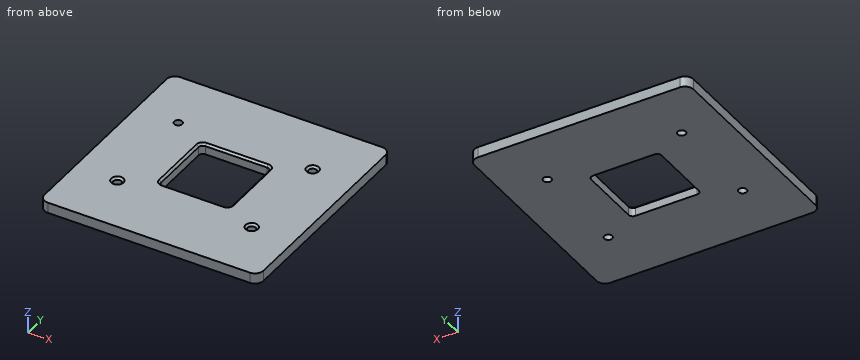
```python
from build123d import *

# Parameters (mm, degrees)
CYLINDER006_R     = 1.9
CYLINDER006_DEPTH = 5
CYLINDER007_R     = 1.9
CYLINDER007_DEPTH = 5
CYLINDER008_R     = 1.9
CYLINDER008_DEPTH = 5
CYLINDER005_R     = 1.9
CYLINDER005_DEPTH = 5
BOX009_W          = 33
BOX009_H          = 33
BOX009_DEPTH      = 5
BOX010_W          = 72
BOX010_H          = 72
BOX010_DEPTH      = 5
FILLET002_R       = 2
FILLET003_R       = 4
CHAMFER001_SIZE   = 1
BOX013_W          = 69.4
BOX013_H          = 69.4
BOX013_DEPTH      = 5
BOX012_W          = 103
BOX012_H          = 103
BOX012_DEPTH      = 5
FILLET005_R       = 4
FILLET006_R       = 2


with BuildPart() as cilindro003:
    # Cylinder006 → Cylinder006 (new body)
    with BuildSketch(Plane(origin=(31.6, 23.7, -48), x_dir=(1, 0, 0), z_dir=(0, 0, 1))):
        Circle(CYLINDER006_R)
    extrude(amount=CYLINDER006_DEPTH)


with BuildPart() as cilindro004:
    # Cylinder007 → Cylinder007 (new body)
    with BuildSketch(Plane(origin=(-31.6, 23.7, -48), x_dir=(1, 0, 0), z_dir=(0, 0, 1))):
        Circle(CYLINDER007_R)
    extrude(amount=CYLINDER007_DEPTH)


with BuildPart() as cilindro005:
    # Cylinder008 → Cylinder008 (new body)
    with BuildSketch(Plane(origin=(-31.6, -23.7, -48), x_dir=(1, 0, 0), z_dir=(0, 0, 1))):
        Circle(CYLINDER008_R)
    extrude(amount=CYLINDER008_DEPTH)


with BuildPart() as compound003:
    # Cylinder005 → Cylinder005 (new body)
    with BuildSketch(Plane(origin=(31.6, -23.7, -48), x_dir=(1, 0, 0), z_dir=(0, 0, 1))):
        Circle(CYLINDER005_R)
    extrude(amount=CYLINDER005_DEPTH)

    # Compound003: union Cilindro003, Cilindro004, Cilindro005
    add(cilindro003.part)
    add(cilindro004.part)
    add(cilindro005.part)


with BuildPart() as cubo008:
    # Box009 → Box009 (new body)
    with BuildSketch(Plane(origin=(-16.5, -16.5, -48), x_dir=(1, 0, 0), z_dir=(0, 0, 1))):
        with Locations((16.5, 16.5)):
            Rectangle(BOX009_W, BOX009_H)
    extrude(amount=BOX009_DEPTH)


with BuildPart() as chamfer001:
    # Box010 → Box010 (new body)
    with BuildSketch(Plane(origin=(-36, -36, -48), x_dir=(1, 0, 0), z_dir=(0, 0, 1))):
        with Locations((36, 36)):
            Rectangle(BOX010_W, BOX010_H)
    extrude(amount=BOX010_DEPTH)

    # Cut003: cut Cubo008
    add(cubo008.part, mode=Mode.SUBTRACT)

    # Fillet002
    fillet002_edges = [chamfer001.edges().sort_by_distance(p)[0] for p in [
        (-16.5, -16.5, -45.5),
        (-16.5, 16.5, -45.5),
        (16.5, -16.5, -45.5),
        (16.5, 16.5, -45.5),
    ]]
    fillet(fillet002_edges, radius=FILLET002_R)

    # Fillet003
    fillet003_edges = [chamfer001.edges().sort_by_distance(p)[0] for p in [
        (-36, -36, -45.5),
        (-36, 36, -45.5),
        (36, 36, -45.5),
        (36, -36, -45.5),
    ]]
    fillet(fillet003_edges, radius=FILLET003_R)

    # Cut006: cut Compound003
    add(compound003.part, mode=Mode.SUBTRACT)

    # Chamfer001
    chamfer001_edges = [chamfer001.edges().sort_by_distance(p)[0] for p in [
        (-33.5, -23.7, -43),
        (29.7, -23.7, -43),
        (-16.5, 0, -43),
        (29.7, 23.7, -43),
    ]]
    chamfer(chamfer001_edges, length=CHAMFER001_SIZE)


with BuildPart() as cubo012:
    # Box013 → Box013 (new body)
    with BuildSketch(Plane(origin=(-34.7, -34.7, -48), x_dir=(1, 0, 0), z_dir=(0, 0, 1))):
        with Locations((34.7, 34.7)):
            Rectangle(BOX013_W, BOX013_H)
    extrude(amount=BOX013_DEPTH)


with BuildPart() as fusion002:
    # Box012 → Box012 (new body)
    with BuildSketch(Plane(origin=(-51.5, -51.5, -48), x_dir=(1, 0, 0), z_dir=(0, 0, 1))):
        with Locations((51.5, 51.5)):
            Rectangle(BOX012_W, BOX012_H)
    extrude(amount=BOX012_DEPTH)

    # Cut005: cut Cubo012
    add(cubo012.part, mode=Mode.SUBTRACT)

    # Fillet005
    fillet005_edges = [fusion002.edges().sort_by_distance(p)[0] for p in [
        (-51.5, -51.5, -45.5),
        (-51.5, 51.5, -45.5),
        (51.5, -51.5, -45.5),
        (51.5, 51.5, -45.5),
    ]]
    fillet(fillet005_edges, radius=FILLET005_R)

    # Fillet006
    fillet006_edges = [fusion002.edges().sort_by_distance(p)[0] for p in [
        (-34.7, -34.7, -45.5),
        (-34.7, 34.7, -45.5),
        (34.7, -34.7, -45.5),
        (34.7, 34.7, -45.5),
    ]]
    fillet(fillet006_edges, radius=FILLET006_R)

    # Fusion002: union Chamfer001
    add(chamfer001.part)


solid = fusion002.part
```
Geometry check sheet. Reference: the model listing, model coordinates, mm. Give positions to 0.01 mm unless a question says otherwise; leave off trailing zeros. Write each loop counter-clockwise with the first axis right and the second up, starting at its lowest first coordinate (ties: lowest second). Pieces come first, ordered by that corner, then holes. Notation, with made-up numbers: (60.5, 12) -> (113.5, 12) arc R24 ccw to (113.5, 35) -> close; hole circle Ø5 at (52.5, 37). An arc over 180 degrees is marked (long way). One line per question, with ' | ' between items.
Item 1: Sectioned sample at B-B, the plane y = 23.7. Record the boundary of the cut face in (x, z), plus the area to 3 significant figures.
Determined:
outline: (-51.5, -48) -> (-33.5, -48) -> (-33.5, -43) -> (-51.5, -43) -> close; (-29.7, -48) -> (29.7, -48) -> (29.7, -44) -> (28.7, -43) -> (-29.7, -43) -> close; (33.5, -48) -> (51.5, -48) -> (51.5, -43) -> (34.5, -43) -> (33.5, -44) -> close | area: 476 mm^2
Item 2: Sectioned sample at A-A, the plane x = 31.6. Record the boundary of the cut face in (y, z), plus the area to 3 significant figures.
Determined:
outline: (-51.5, -48) -> (-25.6, -48) -> (-25.6, -44) -> (-26.6, -43) -> (-51.5, -43) -> close; (-21.8, -48) -> (21.8, -48) -> (21.8, -44) -> (20.8, -43) -> (-20.8, -43) -> (-21.8, -44) -> close; (25.6, -48) -> (51.5, -48) -> (51.5, -43) -> (26.6, -43) -> (25.6, -44) -> close | area: 475 mm^2
Item 3: Scan lines: line 1 along Y through (x, z) = (31.6, -45.15); line 2 along X through (y, z) = (-10.5, -44.6). Record each from-to range of solid material in increasing order.
Determined:
line 1: -51.5 to -25.6, -21.8 to 21.8, 25.6 to 51.5 | line 2: -51.5 to -16.5, 16.5 to 51.5
Item 4: Sectioned sample at C-C, the plane z = -46.75. Record the boundary of the cut face in (x, y).
Determined:
outline: (-51.5, -47.5) arc R4 ccw to (-47.5, -51.5) -> (47.5, -51.5) arc R4 ccw to (51.5, -47.5) -> (51.5, 47.5) arc R4 ccw to (47.5, 51.5) -> (-47.5, 51.5) arc R4 ccw to (-51.5, 47.5) -> close; hole circle Ø3.8 at (-31.6, -23.7); hole circle Ø3.8 at (-31.6, 23.7); hole (-16.5, -14.5) arc R2 ccw to (-14.5, -16.5) -> (14.5, -16.5) arc R2 ccw to (16.5, -14.5) -> (16.5, 14.5) arc R2 ccw to (14.5, 16.5) -> (-14.5, 16.5) arc R2 ccw to (-16.5, 14.5) -> close; hole circle Ø3.8 at (31.6, -23.7); hole circle Ø3.8 at (31.6, 23.7)
Item 5: Sectioned sample at D-D, the plane x = -7. Record the boundary of the cut face in (y, z).
Determined:
outline: (-51.5, -48) -> (-16.5, -48) -> (-16.5, -44) -> (-17.5, -43) -> (-51.5, -43) -> close; (16.5, -48) -> (51.5, -48) -> (51.5, -43) -> (17.5, -43) -> (16.5, -44) -> close
Item 6: Depth check by flat-ended pin: pin 1 (4.5 mm diameter, centred on x = 31.6, y = -23.7, fed in from +Z); pin 2 (4.5 mm diameter, centred on x = 31.6, y = 23.7, fed in from -Z); pin 3 (5 mm diameter, centred on x = -31.6, y = -23.7, fed in from +Z). Enter the tip coordinate at first touch or a pass-through.
Determined:
pin 1: z = -43.65 | pin 2: z = -48 | pin 3: z = -43.4
